The drawing under review shows one solid part. Ordinate dimensions are in mm from its lowest x, y, z. Coordinates: 2 decimals unless noted, no trailing zeros. Loops run counter-clockwise (first coordinate to the right, second up) from the corner with the lowest first, then second, coordinate; pieces in that order, holes last. Notation, with made-up numbers: M 31.5,-37.5 L 48.5,-37.5 A15 ccw 48.5,-28.5 Z; hole C -37.5,33 d10. An arc over 180 degrees is marked long. Put each result on its own line as item: value.
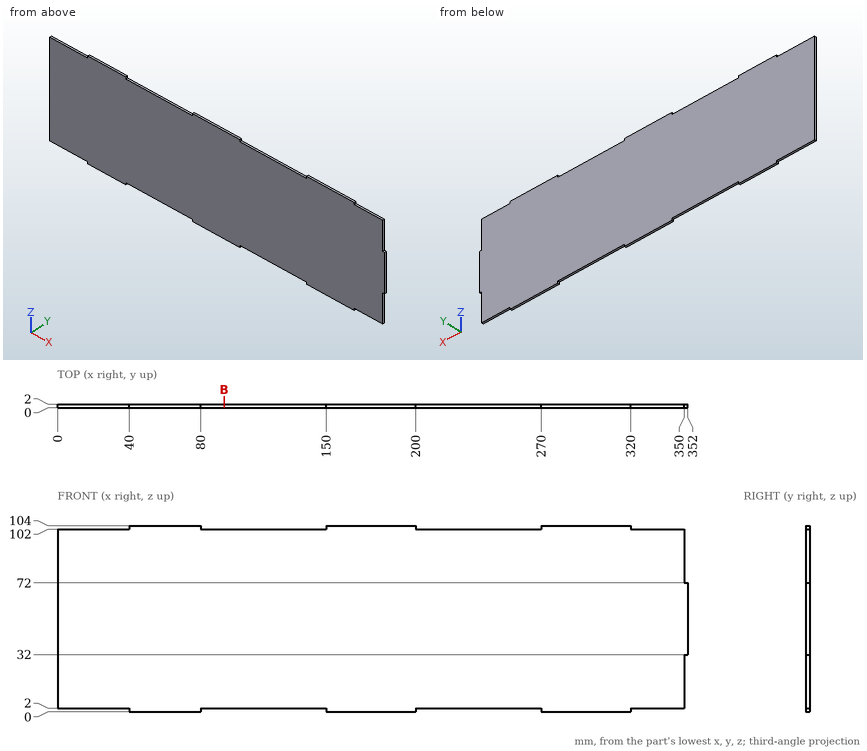
(1) For pin 1 (0.6 mm diameter, centred on y = 1, z = 102.5, fed in from +X); pin 2 (1 mm diameter, centred on x = 231, y = 1, fed in from +Z); pin 3 (1 mm diameter, centred on x = 21, y = 1, fed in from -Z), all flat-tipped, find the tip position at first contact; note any pin that passes through.
Determined:
pin 1: stops at x = 320
pin 2: stops at z = 102
pin 3: stops at z = 2
(2) Wall thickness on line 1 along X through (y, z) = (0.6, 26.5); line 2 along Z through (x, y) = (333.5, 1.8): over which ranges is each line inside the solid? List them lowest first. Write a range as [from, to].
Determined:
line 1: x = [0, 350]
line 2: z = [2, 102]
(3) Add section B-B (x = 93). Write out the cut boundary in (y, z).
Determined:
outline: M 0,2 L 2,2 L 2,102 L 0,102 Z
